Geometry: final body of the model. Coordinates: model frame, mm. Face numbers are marked on the shaded views. A direction names the side the tool comes from. Give positions to 0.01 mm unless a question says otherwise; leave off trailing zeros. Write each loop counter-clockwise with the first axis right and the second up, starting at its lowest first coordinate (ties: lowest second). Pieces come first, ordered by that corner, then holes. Notation, with made-up numbers: (42.25, -14) - (54.25, -14) arc R25 ccw to (54.25, 13) - close; hole circle Ø9 at (84, -29). An arc over 180 degrees is marked (long way). Return JSON: item names as keys, results as strings.
from build123d import *

# Parameters (mm, degrees)
ESQUISSE1_W                  = 78
ESQUISSE1_H                  = 165
BOSS_EXTRU_1_DEPTH           = 250
ENL_V_MAT_EXTRU_1_DEPTH      = 285.020723146
ENL_V_MAT_EXTRU_1_DEPTH_BACK = 78
BOSS_EXTRU_4_START           = 17.177257831
BOSS_EXTRU_4_DEPTH           = 3
BOSS_EXTRU_5_START           = -3
BOSS_EXTRU_5_DEPTH           = 3
BOSS_EXTRU_9_START           = 74
BOSS_EXTRU_9_DEPTH           = 74


# Read off the part's stored shape, not the designer's step: Boss.-Extru.4
with BuildPart() as part:
    # Esquisse1 → Boss.-Extru.1 (new body)
    with BuildSketch(Plane.XY):
        with Locations((-18.822742169, 27.426207869)):
            Rectangle(ESQUISSE1_W, ESQUISSE1_H)
    extrude(amount=BOSS_EXTRU_1_DEPTH)

    # Esquisse2 → Enlèv. mat.-Extru.1 (cut, two sides: drawn at the far end of the back side and taken through both)
    with BuildSketch(Plane.ZY.offset(57.822742169).offset(-ENL_V_MAT_EXTRU_1_DEPTH_BACK)):
        with BuildLine():
            Line((0, -664.156424161), (0, -55.073792131))
            Line((0, -55.073792131), (0, -50.073792131))
            Line((0, -50.073792131), (35, -50.073792131))
            ThreePointArc((35, -50.073792131), (165.813798966, -5.411019544), (242, 109.926207869))
            Line((242, 109.926207869), (395.487506317, 699.35240176))
            Line((395.487506317, 699.35240176), (-774.457853053, 1038.696573142))
            Line((-774.457853053, 1038.696573142), (-1169.94535937, -324.812252779))
            Line((-1169.94535937, -324.812252779), (0, -664.156424161))
        make_face()
    extrude(amount=ENL_V_MAT_EXTRU_1_DEPTH + ENL_V_MAT_EXTRU_1_DEPTH_BACK, mode=Mode.SUBTRACT)

    # Boss.-Extru.4 outline → Boss.-Extru.4 (add)
    with BuildSketch(Plane.YZ.offset(BOSS_EXTRU_4_START)):
        with BuildLine():
            Line((-50.073792131, 0), (21.926207869, 0))
            Line((21.926207869, 0), (21.926207869, 33.303690661))
            ThreePointArc((21.926207869, 33.303690661), (43.150814353, 104.129560556), (87.912843237, 162.978082516))
            Line((87.912843237, 162.978082516), (87.912843237, 234.978082516))
            ThreePointArc((87.912843237, 234.978082516), (-12.229352313, 156.482040882), (-50.073792131, 35))
            Line((-50.073792131, 35), (-50.073792131, 0))
        make_face()
    extrude(amount=BOSS_EXTRU_4_DEPTH)

    # Esquisse7 → Boss.-Extru.5 (add)
    with BuildSketch(Plane.ZY.offset(57.822742169).offset(BOSS_EXTRU_5_START)):
        with BuildLine():
            Line((0, -50.073792131), (0, 21.926207869))
            Line((0, 21.926207869), (33.3, 21.926207869))
            ThreePointArc((33.3, 21.926207869), (104.127859837, 43.15019521), (162.978082516, 87.912843237))
            Line((162.978082516, 87.912843237), (234.978082516, 87.912843237))
            ThreePointArc((234.978082516, 87.912843237), (156.482040881, -12.229352313), (35, -50.073792131))
            Line((35, -50.073792131), (0, -50.073792131))
        make_face()
    extrude(amount=BOSS_EXTRU_5_DEPTH)

    # Esquisse22 → Boss.-Extru.9 (add)
    with BuildSketch(Plane(origin=(-54.822742169, 0, 0), x_dir=(0, 0, -1), z_dir=(1, 0, 0)).offset(BOSS_EXTRU_9_START)):
        with BuildLine():
            Line((-33.3, 21.926207869), (-33.3, 19.926207869))
            ThreePointArc((-33.3, 19.926207869), (-105.482114961, 41.634114192), (-164.978082516, 87.912843237))
            Line((-164.978082516, 87.912843237), (-162.978082516, 87.912843237))
            ThreePointArc((-162.978082516, 87.912843237), (-104.127859837, 43.15019521), (-33.3, 21.926207869))
        make_face()
    extrude(amount=-BOSS_EXTRU_9_DEPTH)


solid = part.part
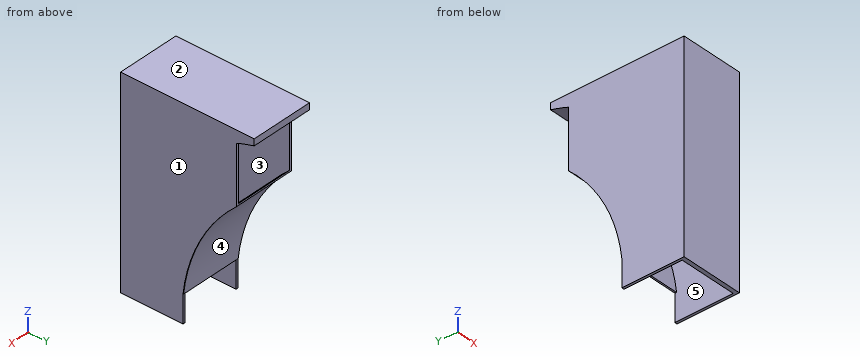
Q1. Section query A-A, the plane x = -9. Return the cut outline in (y, z).
Answer key:
{"outline": "(-55.07, 0) - (-50.07, 0) - (-50.07, 35) arc R213.9 cw to (109.93, 242) - (109.93, 250) - (-55.07, 250) - close; (19.93, 33.3) - (21.93, 33.3) arc R207 cw to (87.91, 162.98) - (87.91, 164.98) arc R205.46 ccw to start"}
Q2. Mould query, pull axis X, two halves, no side actions, for the marked faces 1, 2 and 3. Classes: pulls with the +X half, pulls with the -X half, needs draft (parallel to the pull), parting line crosses it, or undercut.
Answer key:
{"face 1": "pulls with the +X half", "face 2": "needs draft", "face 3": "undercut"}
Q3. Section query B-B, the plane z = 17. Return the cut outline in (x, y).
Answer key:
{"outline": "(-57.82, -55.07) - (20.18, -55.07) - (20.18, 21.93) - (17.18, 21.93) - (17.18, -50.07) - (-54.82, -50.07) - (-54.82, 21.93) - (-57.82, 21.93) - close"}
Q4. Material intervals for probe 1 along X at (y, z) = (-20.5, 18.5); probe 2 along Y at (x, z) = (-6, 126); probe 3 along Z at (x, y) = (-17.5, 57), sorted ascending. Write a range as [from, to].
Answer key:
{"probe 1": "x = [-57.82, -54.82], [17.18, 20.18]", "probe 2": "y = [-55.07, -29.75], [53.79, 56.03]", "probe 3": "z = [127.43, 130.63], [220.32, 250]"}
Q5. Set-up query: the marked faces 4 and 5. Return all of +Z, -Z, +X, -X, +Y, -Y with unobstructed straight access to the full face (end or side cutting, diameter ignored); none if empty.
Answer key:
{"face 4": "-Z, +X, -X, +Y", "face 5": "none"}
Q6. Pin query (flat end, axial travel): P1, Ø1, axis at x = -21, y = 21, coming from the -Z side; P2, Ø17.5, axis at x = -30.5, z = 21, coming from the +Y side; P3, Ø0.9, axis at x = -56, z = 18, coming from the +Y side. Return the tip coordinate at first contact, or that it passes through.
Answer key:
{"P1": "stops at z = 33.3", "P2": "stops at y = -50.07", "P3": "stops at y = 21.93"}
